Can you work these out from the model? Positions are in its coordinate system, mm. Face numbers are marked on the shaded views. Give positions to 0.01 mm unless a question says otherwise; leave off trailing zeros. Write each loop counter-clockwise with the first axis right and the second up, starting at its lowest first coordinate (ties: lowest second). Pieces come first, ordered by that corner, then holes. Notation, with made-up numbers: (28.25, 29.25) - (44.25, 29.25) arc R17 ccw to (44.25, 61.25) - close; hole circle Ø11 at (-21, 83). An arc over 180 degrees is marked (long way). Use a Markdown table: item, result. Add a question column.
```python
from build123d import *

# Parameters (mm, degrees)
SZKIC1_W                                  = 237
SZKIC1_H                                  = 145
DODANIE_WYCI_GNI_CIE1_DEPTH               = 5
SZKIC2_W                                  = 7
SZKIC2_H                                  = 135
DODANIE_WYCI_GNI_CIE2_DEPTH               = 10
OTW_R_4_0_4_1_D                           = 4
OTW_R_4_0_4_1_DEPTH                       = 6.7
SFAZOWANIE1_SIZE                          = 10
WYTNIJ_WYCI_GNI_CIE1_REACH                = 141.727
SZKIC5_W                                  = 30
SZKIC5_H                                  = 6
POG_BIENIE_WALCOWE_POD_M3_RUB_Z_B_2_COUNT = 2
POG_BIENIE_WALCOWE_POD_M3_RUB_Z_B_2_PITCH = 75
POG_BIENIE_WALCOWE_POD_M3_RUB_Z_B_3_COUNT = 2
POG_BIENIE_WALCOWE_POD_M3_RUB_Z_B_3_PITCH = 154.2


with BuildPart() as part:
    # Szkic1 → Dodanie-wyciągnięcie1 (new body)
    with BuildSketch(Plane.XY):
        Rectangle(SZKIC1_W, SZKIC1_H)
    extrude(amount=DODANIE_WYCI_GNI_CIE1_DEPTH)

    # Szkic2 → Dodanie-wyciągnięcie2 (add)
    with BuildSketch(Plane.XY.offset(5)):
        with Locations((115, -5)):
            Rectangle(SZKIC2_W, SZKIC2_H)
        with Locations((-115, -5)):
            Rectangle(SZKIC2_W, SZKIC2_H)
    extrude(amount=DODANIE_WYCI_GNI_CIE2_DEPTH)

    # Otwór Ø4.0 (4)1
    with Locations(Plane(origin=(118.5, 0, 0), x_dir=(0, 0, -1), z_dir=(1, 0, 0))):
        with Locations((-10, -42.5), (-10, 32.5), (-10, -5)):
            otw_r_4_0_4_1 = Hole(OTW_R_4_0_4_1_D / 2, depth=OTW_R_4_0_4_1_DEPTH)

    # Lustro1: Otwór Ø4.0 (4)1 across plane
    add(otw_r_4_0_4_1.mirror(Plane.ZY), mode=Mode.SUBTRACT)

    # Sfazowanie1
    sfazowanie1_edges = [part.edges().sort_by_distance(p)[0] for p in [
        (-115, 62.5, 15),
        (115, 62.5, 15),
    ]]
    chamfer(sfazowanie1_edges, length=SFAZOWANIE1_SIZE - 0.0001)  # a hair under: the kernel refuses the full size

    # Szkic5 → Wytnij-wyciągnięcie1 (cut, up to next)
    with BuildSketch(Plane(origin=(0, 0, 0), x_dir=(-1, 0, 0), z_dir=(0, 0, -1)), mode=Mode.PRIVATE) as wytnij_wyci_gni_cie1_sk1:
        with Locations((-99.5, 69.5)):
            Rectangle(SZKIC5_W, SZKIC5_H)
    wytnij_wyci_gni_cie1_tool1 = extrude(wytnij_wyci_gni_cie1_sk1.sketch, amount=-WYTNIJ_WYCI_GNI_CIE1_REACH, mode=Mode.PRIVATE) & part.part
    # Szkic5 → Wytnij-wyciągnięcie1 (cut, up to next)
    with BuildSketch(Plane(origin=(0, 0, 0), x_dir=(-1, 0, 0), z_dir=(0, 0, -1)), mode=Mode.PRIVATE) as wytnij_wyci_gni_cie1_sk2:
        Polygon((-84.1, 72.5), (-84.5, 72.5), (-84.5, 66.5), (-114.5, 66.5), (-114.5, 72.5), (-114.9, 72.5), (-114.9, 66.1), (-84.1, 66.1), align=None)
    wytnij_wyci_gni_cie1_tool2 = extrude(wytnij_wyci_gni_cie1_sk2.sketch, amount=-WYTNIJ_WYCI_GNI_CIE1_REACH, mode=Mode.PRIVATE) & part.part
    # Szkic5 → Wytnij-wyciągnięcie1 (cut, up to next)
    with BuildSketch(Plane(origin=(0, 0, 0), x_dir=(-1, 0, 0), z_dir=(0, 0, -1)), mode=Mode.PRIVATE) as wytnij_wyci_gni_cie1_sk3:
        Polygon((-89.4, 62.9), (-89.4, 42.154636006), (-86.220321431, 42.154636006), (-85.282842712, 41.217157288), (-82.4, 38.334314575), (-82.4, 8.1), (-41.6, 8.1), (-41.6, 38.334314575), (-38.717157288, 41.217157288), (-37.779678569, 42.154636006), (-34.6, 42.154636006), (-34.6, 62.9), align=None)
        Polygon((-42, 8.5), (-42, 38.5), (-39, 41.5), (-38, 42.5), (-38, 42.554636006), (-35, 42.554636006), (-35, 62.5), (-89, 62.5), (-89, 42.554636006), (-86, 42.554636006), (-86, 42.5), (-85, 41.5), (-82, 38.5), (-82, 8.5), align=None, mode=Mode.SUBTRACT)
    wytnij_wyci_gni_cie1_tool3 = extrude(wytnij_wyci_gni_cie1_sk3.sketch, amount=-WYTNIJ_WYCI_GNI_CIE1_REACH, mode=Mode.PRIVATE) & part.part
    # Szkic5 → Wytnij-wyciągnięcie1 (cut, up to next)
    with BuildSketch(Plane(origin=(0, 0, 0), x_dir=(-1, 0, 0), z_dir=(0, 0, -1)), mode=Mode.PRIVATE) as wytnij_wyci_gni_cie1_sk4:
        Polygon((-82, 8.5), (-42, 8.5), (-42, 38.5), (-39, 41.5), (-38, 42.5), (-38, 42.554636006), (-35, 42.554636006), (-35, 62.5), (-89, 62.5), (-89, 42.554636006), (-86, 42.554636006), (-86, 42.5), (-85, 41.5), (-82, 38.5), align=None)
    wytnij_wyci_gni_cie1_tool4 = extrude(wytnij_wyci_gni_cie1_sk4.sketch, amount=-WYTNIJ_WYCI_GNI_CIE1_REACH, mode=Mode.PRIVATE) & part.part
    # Szkic5 → Wytnij-wyciągnięcie1 (cut, up to next)
    with BuildSketch(Plane(origin=(0, 0, 0), x_dir=(-1, 0, 0), z_dir=(0, 0, -1)), mode=Mode.PRIVATE) as wytnij_wyci_gni_cie1_sk5:
        Polygon((-14.4, 62.9), (-14.4, 42.154636006), (-11.220321431, 42.154636006), (-10.282842712, 41.217157288), (-7.4, 38.334314575), (-7.4, 8.1), (33.4, 8.1), (33.4, 38.334314575), (36.282842712, 41.217157288), (37.220321431, 42.154636006), (40.4, 42.154636006), (40.4, 62.9), align=None)
        Polygon((33, 8.5), (33, 38.5), (36, 41.5), (37, 42.5), (37, 42.554636006), (40, 42.554636006), (40, 62.5), (-14, 62.5), (-14, 42.554636006), (-11, 42.554636006), (-11, 42.5), (-10, 41.5), (-7, 38.5), (-7, 8.5), align=None, mode=Mode.SUBTRACT)
    wytnij_wyci_gni_cie1_tool5 = extrude(wytnij_wyci_gni_cie1_sk5.sketch, amount=-WYTNIJ_WYCI_GNI_CIE1_REACH, mode=Mode.PRIVATE) & part.part
    # Szkic5 → Wytnij-wyciągnięcie1 (cut, up to next)
    with BuildSketch(Plane(origin=(0, 0, 0), x_dir=(-1, 0, 0), z_dir=(0, 0, -1)), mode=Mode.PRIVATE) as wytnij_wyci_gni_cie1_sk6:
        Polygon((-7, 8.5), (33, 8.5), (33, 38.5), (36, 41.5), (37, 42.5), (37, 42.554636006), (40, 42.554636006), (40, 62.5), (-14, 62.5), (-14, 42.554636006), (-11, 42.554636006), (-11, 42.5), (-10, 41.5), (-7, 38.5), align=None)
    wytnij_wyci_gni_cie1_tool6 = extrude(wytnij_wyci_gni_cie1_sk6.sketch, amount=-WYTNIJ_WYCI_GNI_CIE1_REACH, mode=Mode.PRIVATE) & part.part
    # Szkic5 → Wytnij-wyciągnięcie1 (cut, up to next)
    with BuildSketch(Plane(origin=(0, 0, 0), x_dir=(-1, 0, 0), z_dir=(0, 0, -1)), mode=Mode.PRIVATE) as wytnij_wyci_gni_cie1_sk7:
        with Locations((-24.5, 69.5)):
            Rectangle(SZKIC5_W, SZKIC5_H)
    wytnij_wyci_gni_cie1_tool7 = extrude(wytnij_wyci_gni_cie1_sk7.sketch, amount=-WYTNIJ_WYCI_GNI_CIE1_REACH, mode=Mode.PRIVATE) & part.part
    # Szkic5 → Wytnij-wyciągnięcie1 (cut, up to next)
    with BuildSketch(Plane(origin=(0, 0, 0), x_dir=(-1, 0, 0), z_dir=(0, 0, -1)), mode=Mode.PRIVATE) as wytnij_wyci_gni_cie1_sk8:
        Polygon((-39.5, 72.5), (-39.9, 72.5), (-39.9, 66.1), (-9.1, 66.1), (-9.1, 72.5), (-9.5, 72.5), (-9.5, 66.5), (-39.5, 66.5), align=None)
    wytnij_wyci_gni_cie1_tool8 = extrude(wytnij_wyci_gni_cie1_sk8.sketch, amount=-WYTNIJ_WYCI_GNI_CIE1_REACH, mode=Mode.PRIVATE) & part.part
    # Szkic5 → Wytnij-wyciągnięcie1 (cut, up to next)
    with BuildSketch(Plane(origin=(0, 0, 0), x_dir=(-1, 0, 0), z_dir=(0, 0, -1)), mode=Mode.PRIVATE) as wytnij_wyci_gni_cie1_sk9:
        Polygon((60.6, 62.9), (60.6, 42.154636006), (63.779678569, 42.154636006), (64.717157288, 41.217157288), (67.6, 38.334314575), (67.6, 8.1), (108.4, 8.1), (108.4, 38.334314575), (111.282842712, 41.217157288), (112.220321431, 42.154636006), (115.4, 42.154636006), (115.4, 62.9), align=None)
        Polygon((108, 8.5), (108, 38.5), (111, 41.5), (112, 42.5), (112, 42.554636006), (115, 42.554636006), (115, 62.5), (61, 62.5), (61, 42.554636006), (64, 42.554636006), (64, 42.5), (65, 41.5), (68, 38.5), (68, 8.5), align=None, mode=Mode.SUBTRACT)
    wytnij_wyci_gni_cie1_tool9 = extrude(wytnij_wyci_gni_cie1_sk9.sketch, amount=-WYTNIJ_WYCI_GNI_CIE1_REACH, mode=Mode.PRIVATE) & part.part
    # Szkic5 → Wytnij-wyciągnięcie1 (cut, up to next)
    with BuildSketch(Plane(origin=(0, 0, 0), x_dir=(-1, 0, 0), z_dir=(0, 0, -1)), mode=Mode.PRIVATE) as wytnij_wyci_gni_cie1_sk10:
        Polygon((68, 8.5), (108, 8.5), (108, 38.5), (111, 41.5), (112, 42.5), (112, 42.554636006), (115, 42.554636006), (115, 62.5), (61, 62.5), (61, 42.554636006), (64, 42.554636006), (64, 42.5), (65, 41.5), (68, 38.5), align=None)
    wytnij_wyci_gni_cie1_tool10 = extrude(wytnij_wyci_gni_cie1_sk10.sketch, amount=-WYTNIJ_WYCI_GNI_CIE1_REACH, mode=Mode.PRIVATE) & part.part
    # Szkic5 → Wytnij-wyciągnięcie1 (cut, up to next)
    with BuildSketch(Plane(origin=(0, 0, 0), x_dir=(-1, 0, 0), z_dir=(0, 0, -1)), mode=Mode.PRIVATE) as wytnij_wyci_gni_cie1_sk11:
        with Locations((50.5, 69.5)):
            Rectangle(SZKIC5_W, SZKIC5_H)
    wytnij_wyci_gni_cie1_tool11 = extrude(wytnij_wyci_gni_cie1_sk11.sketch, amount=-WYTNIJ_WYCI_GNI_CIE1_REACH, mode=Mode.PRIVATE) & part.part
    # Szkic5 → Wytnij-wyciągnięcie1 (cut, up to next)
    with BuildSketch(Plane(origin=(0, 0, 0), x_dir=(-1, 0, 0), z_dir=(0, 0, -1)), mode=Mode.PRIVATE) as wytnij_wyci_gni_cie1_sk12:
        Polygon((35.5, 72.5), (35.1, 72.5), (35.1, 66.1), (65.9, 66.1), (65.9, 72.5), (65.5, 72.5), (65.5, 66.5), (35.5, 66.5), align=None)
    wytnij_wyci_gni_cie1_tool12 = extrude(wytnij_wyci_gni_cie1_sk12.sketch, amount=-WYTNIJ_WYCI_GNI_CIE1_REACH, mode=Mode.PRIVATE) & part.part
    add(wytnij_wyci_gni_cie1_tool1.solids().sort_by_distance((99.5, 69.5, 0))[0], mode=Mode.SUBTRACT)
    add(wytnij_wyci_gni_cie1_tool2.solids().sort_by_distance((84.3, 72.185421, 0))[0], mode=Mode.SUBTRACT)
    add(wytnij_wyci_gni_cie1_tool3.solids().sort_by_distance((89.322501, 52.527318, 0))[0], mode=Mode.SUBTRACT)
    add(wytnij_wyci_gni_cie1_tool4.solids().sort_by_distance((62, 37.474353, 0))[0], mode=Mode.SUBTRACT)
    add(wytnij_wyci_gni_cie1_tool5.solids().sort_by_distance((14.322501, 52.527318, 0))[0], mode=Mode.SUBTRACT)
    add(wytnij_wyci_gni_cie1_tool6.solids().sort_by_distance((-13, 37.474353, 0))[0], mode=Mode.SUBTRACT)
    add(wytnij_wyci_gni_cie1_tool7.solids().sort_by_distance((24.5, 69.5, 0))[0], mode=Mode.SUBTRACT)
    add(wytnij_wyci_gni_cie1_tool8.solids().sort_by_distance((39.7, 72.185421, 0))[0], mode=Mode.SUBTRACT)
    add(wytnij_wyci_gni_cie1_tool9.solids().sort_by_distance((-60.677499, 52.527318, 0))[0], mode=Mode.SUBTRACT)
    add(wytnij_wyci_gni_cie1_tool10.solids().sort_by_distance((-88, 37.474353, 0))[0], mode=Mode.SUBTRACT)
    add(wytnij_wyci_gni_cie1_tool11.solids().sort_by_distance((-50.5, 69.5, 0))[0], mode=Mode.SUBTRACT)
    add(wytnij_wyci_gni_cie1_tool12.solids().sort_by_distance((-65.814579, 69.5, 0))[0], mode=Mode.SUBTRACT)


with BuildPart() as body_2:
    # Podziel1: the piece on the far side of the plane
    add(part.part)
    split(bisect_by=Plane(origin=(0, -22.5, 0), x_dir=(0, 0, -1), z_dir=(0, -1, 0)), keep=Keep.BOTTOM)

    # Szkic7 → Pogłębienie walcowe pod M3 Śrubę z łbem stożkowym ściętym1 (revolve, cut)
    with BuildSketch(Plane(origin=(62, 67.5, 0), x_dir=(0, 1, 0), z_dir=(1, 0, 0))):
        Polygon((0, 0), (0, 7.781549114), (1.8, 6.7), (1.8, 2.4), (3.5, 2.4), (3.5, 0), align=None)
    pog_bienie_walcowe_pod_m3_rub_z_bem_s = revolve(axis=Axis((62, 67.5, -6.35), (0, 0, 1)), mode=Mode.SUBTRACT)

    # Pog_bienie walcowe pod M3 _rub_ z _b 2: Pogłębienie walcowe pod M3 Śrubę z łbem stożkowym ściętym1 ×2
    with Locations(*[(-i * POG_BIENIE_WALCOWE_POD_M3_RUB_Z_B_2_PITCH, 0, 0) for i in range(1, POG_BIENIE_WALCOWE_POD_M3_RUB_Z_B_2_COUNT)]):
        add(pog_bienie_walcowe_pod_m3_rub_z_bem_s, mode=Mode.SUBTRACT)

    # Pog_bienie walcowe pod M3 _rub_ z _b 3: Pogłębienie walcowe pod M3 Śrubę z łbem stożkowym ściętym1 ×2
    with Locations(*[(-i * POG_BIENIE_WALCOWE_POD_M3_RUB_Z_B_3_PITCH, 0, 0) for i in range(1, POG_BIENIE_WALCOWE_POD_M3_RUB_Z_B_3_COUNT)]):
        add(pog_bienie_walcowe_pod_m3_rub_z_bem_s, mode=Mode.SUBTRACT)


with BuildPart() as part_1:
    add(part.part)

    # Podziel1
    split(bisect_by=Plane(origin=(0, -22.5, 0), x_dir=(0, 0, -1), z_dir=(0, -1, 0)), keep=Keep.TOP)


solid = body_2.part
```
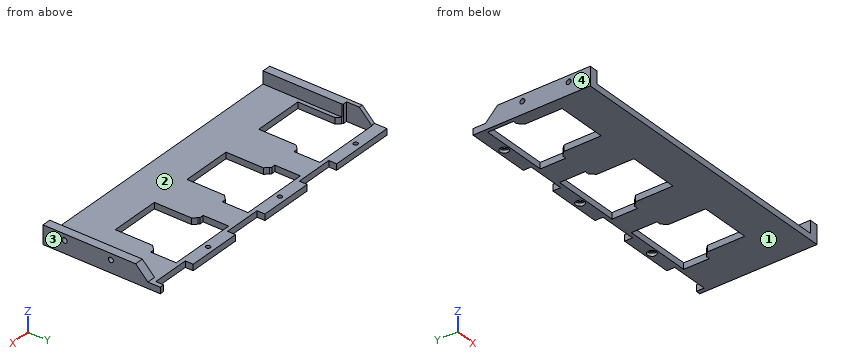
Q1. I'm going to push flat-ended pins straight in: P1, Ø3.5, axis at y = -5, z = 10, coming from the -X side; P2, Ø4.5, axis at y = 32.5, z = 10, coming from the +X side; P3, Ø4, axis at x = 62, y = 67.5, coming from the +Z side. Where does each tip first touch, or does it pass through?
Q2. If we mould it in two halves opening along X, with no side actions, what happens to the marked faces 1, 2, 3 and 4? For each: released by +X, released by -X, zero draft, split by the parting line, or undercut.
Q3. If I drill on probe 1 along Y at (x, z) = (-113.75, 10); probe 2 along X at (y, z) = (33.5, 1.25); probe 3 along Y at (x, z) = (-13, 3.6), over which ranges is the centre line in solid material (lowest first)? Write a range as [from, to].
Q4. Suppose I cut it at A-A (y = 26). Please give me the cut outline in (x, z), and give its area (3 significant figures).
Q5. Suppose I cut it at C-C (y = -12). Please give me the cut outline in (x, z), and give its area (4 significant figures).
Q6. Suppose I cut it at B-B (x = 78). Please give me the cut outline in (y, z).
Q7. Suppose I cut it at D-D (x = 28). Please give me the cut outline in (y, z).
Derived:
| question | item | result |
|---|---|---|
| 1 | P1 | x = -111.8 |
| 1 | P2 | x = 118.5 |
| 1 | P3 | z = 5 |
| 2 | face 1 | zero draft |
| 2 | face 2 | undercut |
| 2 | face 3 | released by +X |
| 2 | face 4 | released by -X |
| 3 | probe 1 | [-22.5, -7], [-3, 30.5], [34.5, 42.15] |
| 3 | probe 2 | [-118.5, -108.4], [-67.6, -33.4], [7.4, 41.6], [82.4, 118.5] |
| 3 | probe 3 | [-22.5, 8.1], [62.9, 65.7], [69.3, 72.5] |
| 4 | outline | (-118.5, 0) - (-108.4, 0) - (-108.4, 5) - (-111.5, 5) - (-111.5, 15) - (-118.5, 15) - close; (-67.6, 0) - (-33.4, 0) - (-33.4, 5) - (-67.6, 5) - close; (7.4, 0) - (41.6, 0) - (41.6, 5) - (7.4, 5) - close; (82.4, 0) - (118.5, 0) - (118.5, 15) - (111.5, 15) - (111.5, 5) - (82.4, 5) - close |
| 4 | area | 713 mm² |
| 5 | outline | (-118.5, 0) - (118.5, 0) - (118.5, 15) - (111.5, 15) - (111.5, 5) - (-111.5, 5) - (-111.5, 15) - (-118.5, 15) - close |
| 5 | area | 1,325 mm² |
| 6 | outline | (-22.5, 0) - (8.1, 0) - (8.1, 5) - (-22.5, 5) - close; (62.9, 0) - (72.5, 0) - (72.5, 5) - (62.9, 5) - close |
| 7 | outline | (-22.5, 0) - (66.1, 0) - (66.1, 5) - (-22.5, 5) - close |
